```python
from build123d import *

# Parameters (mm, degrees)
SKETCH1_W           = 88
SKETCH1_H           = 55
BOSS_EXTRUDE1_DEPTH = 18
BOSS_EXTRUDE2_DEPTH = 38
CUT_EXTRUDE4_DEPTH  = 38


with BuildPart() as part:
    # Sketch1 → Boss-Extrude1 (new body)
    with BuildSketch(Plane(origin=(0, 0, 0), x_dir=(1, 0, 0), z_dir=(0, 1, 0))):
        Rectangle(SKETCH1_W, SKETCH1_H)
    extrude(amount=BOSS_EXTRUDE1_DEPTH)

    # Sketch2 → Boss-Extrude2 (add)
    with BuildSketch(Plane(origin=(0, 18, 0), x_dir=(1, 0, 0), z_dir=(0, 1, 0))):
        Polygon((-6, 27.5), (-6, 12.5), (-44, 12.5), (-44, 0.5), (-6, 0.5), (-6, -27.5), (6, -27.5), (6, 0.5), (44, 0.5), (44, 12.5), (6, 12.5), (6, 27.5), align=None)
    extrude(amount=BOSS_EXTRUDE2_DEPTH)

    # Sketch6 → Cut-Extrude4 (cut)
    with BuildSketch(Plane(origin=(23.709993468, 23.709993468, 24.141084259), x_dir=(-0.8189594221707254, 0.4021022970404831, 0.4094132478957647), z_dir=(-0.5738514309799984, -0.5738514309800047, -0.5842850933614594))):
        Polygon((-24.775350258, -19.269470409), (43.604106017, 20.683626585), (-24.775350258, 59.222567403), align=None)
    extrude(amount=-CUT_EXTRUDE4_DEPTH, mode=Mode.SUBTRACT)


solid = part.part
```
Check sheet for the modelled part. Datum: model origin and axes. Units: mm. A direction names the side the tool comes from. Give positions to 0.01 mm unless a question says otherwise; leave off trailing zeros. Loops run counter-clockwise (first coordinate to the right, second up) from the corner with the lowest first, then second, coordinate; pieces in that order, holes last. Notation, with made-up numbers: (67, -29) - (72, -29) arc R9 ccw to (72, -12) - close; hole circle Ø1 at (-23, 23.5). An arc over 180 degrees is marked (long way). One line per question, with ' | ' between items. Start each with the question number.
1. Set-up check for faces 1 (the flat face through (-25, 37, -12.5)), 2 (the flat face through (6, 37, -20)), 3 (the flat face through (21, 18, 13)), 4 (the flat face through (-6, 37, 13)): record each of +Z, -Z, +X, -X, +Y, -Y from which the full face is reachable in a straight line by a thin tool's end or side.
2. Material ranges on line 1 along Y through (x, z) = (18, -21); line 2 along Z through (x, y) = (21, 33.5); line 3 along X through (y, z) = (45, -21.5), recorded low to high. Write a range as [from, to].
3. Cross-section at A-A, the plane y = 22.5. Enter the section's corners in (x, z), plus the area to 3 significant figures.
4. Gauge pin test, flat ends, axial feed: pin 1 Ø14 at (x, z) = (-32, 9.5) entering from +Y; pin 2 Ø5 at (x, y) = (10.5, 41) entering from -Z; pin 3 Ø4.5 at (y, z) = (42, -19.5) entering from +X; pin 4 Ø16.5 at (y, z) = (42, -19) entering from -X. Record the tip position at first contact, or that the pin passes through.
5. Cross-section at D-D, the plane z = 18. Enter the section's corners in (x, y).
6. Cross-section at B-B, the plane z = 6. Enter the section's corners in (x, y), plus the area to 3 significant figures.
7. Cross-section at C-C, the plane x = -25.5. Enter the section's corners in (y, z).
Check result:
1) face 1: -Z, -X, +Y | face 2: -Z, +X, +Y | face 3: +Z, +X, +Y | face 4: +Z, -X, +Y
2) line 1: y = [0, 18] | line 2: z = [-12.5, -0.5] | line 3: x = [-6, 6]
3) outline: (-44, -12.5) - (-6, -12.5) - (-6, -27.5) - (6, -27.5) - (6, -12.5) - (44, -12.5) - (44, -0.5) - (6, -0.5) - (6, 27.5) - (-6, 27.5) - (-6, -0.5) - (-44, -0.5) - close | area: 1,570 mm2
4) pin 1: stops at y = 18 | pin 2: stops at z = -12.5 | pin 3: stops at x = 6 | pin 4: stops at x = -44
5) outline: (-44, 0) - (44, 0) - (44, 9.67) - (35.67, 18) - (6, 18) - (6, 47.67) - (-2.33, 56) - (-6, 56) - (-6, 18) - (-44, 18) - close
6) outline: (-44, 0) - (44, 0) - (44, 18) - (6, 18) - (6, 56) - (-6, 56) - (-6, 18) - (-44, 18) - close | area: 2,040 mm2
7) outline: (0, -27.5) - (18, -27.5) - (18, -12.5) - (56, -12.5) - (56, -0.5) - (18, -0.5) - (18, 27.5) - (0, 27.5) - close
